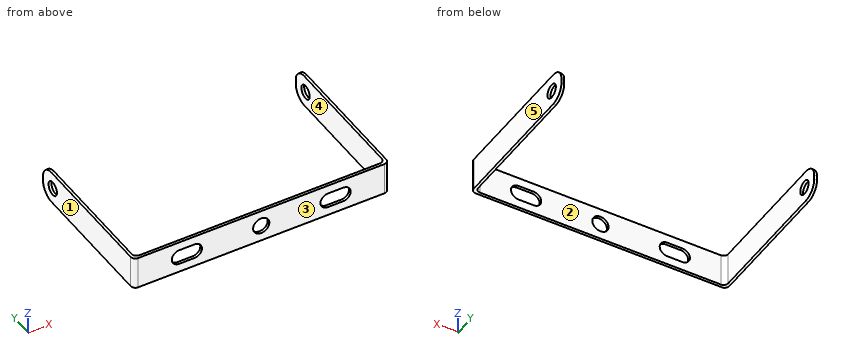
```python
from build123d import *

# Parameters (mm, degrees)
AUFSATZ_LINEAR_AUSTRAGEN1_DEPTH = 14
VERRUNDUNG1_R                   = 2
SKIZZE2_R                       = 3
SCHNITT_LINEAR_AUSTRAGEN1_DEPTH = 129.534042183
VERRUNDUNG2_R                   = 6
SKIZZE3_R                       = 3.5
SCHNITT_LINEAR_AUSTRAGEN2_DEPTH = 129.534042183


with BuildPart() as part:
    # Skizze1 → Aufsatz-Linear austragen1 (new body)
    with BuildSketch(Plane.XY):
        Polygon((0, 0), (-110, 0), (-110, 65), (-108.8, 65), (-108.8, 1.2), (-1.2, 1.2), (-1.2, 65), (0, 65), align=None)
    extrude(amount=AUFSATZ_LINEAR_AUSTRAGEN1_DEPTH)

    # Verrundung1
    verrundung1_edges = [part.edges().sort_by_distance(p)[0] for p in [
        (0, 0, 7),
        (-110, 0, 7),
        (-108.8, 1.2, 7),
        (-1.2, 1.2, 7),
    ]]
    fillet(verrundung1_edges, radius=VERRUNDUNG1_R)

    # Skizze2 → Schnitt-Linear austragen1 (cut, through all)
    with BuildSketch(Plane(origin=(0, 0, 0), x_dir=(0, 0, -1), z_dir=(1, 0, 0))):
        with Locations((-7, 58)):
            Circle(SKIZZE2_R)
    extrude(amount=-SCHNITT_LINEAR_AUSTRAGEN1_DEPTH, mode=Mode.SUBTRACT)

    # Verrundung2
    verrundung2_edges = [part.edges().sort_by_distance(p)[0] for p in [
        (-0.6, 65, 0),
        (-109.4, 65, 14),
        (-0.6, 65, 14),
        (-109.4, 65, 0),
    ]]
    fillet(verrundung2_edges, radius=VERRUNDUNG2_R)

    # Skizze3 → Schnitt-Linear austragen2 (cut, through all)
    with BuildSketch(Plane(origin=(0, 0, 0), x_dir=(-1, 0, 0), z_dir=(0, -1, 0))):
        with Locations(Location((55, -7, 0), (0, 0, 90))):
            Circle(SKIZZE3_R)
        with BuildLine():
            Line((90.25, -10.25), (83.75, -10.25))
            ThreePointArc((83.75, -10.25), (80.5, -7), (83.75, -3.75))
            Line((83.75, -3.75), (90.25, -3.75))
            ThreePointArc((90.25, -3.75), (93.5, -7), (90.25, -10.25))
        make_face()
        with BuildLine():
            Line((19.75, -10.25), (26.25, -10.25))
            ThreePointArc((26.25, -10.25), (29.5, -7), (26.25, -3.75))
            Line((26.25, -3.75), (19.75, -3.75))
            ThreePointArc((19.75, -3.75), (16.5, -7), (19.75, -10.25))
        make_face()
    extrude(amount=-SCHNITT_LINEAR_AUSTRAGEN2_DEPTH, mode=Mode.SUBTRACT)


solid = part.part
```
Verification items for the finished model (mm, model axes). Face numbers are marked on the shaded views. A direction names the side the tool comes from. Round coordinates to 2 decimals unless told otherwise and drop trailing zeros. Write each loop counter-clockwise with the first axis right and the second up, starting at its lowest first coordinate (ties: lowest second). Pieces come first, ordered by that corner, then holes.
1. Gauge pin test, flat ends, axial feed: P1, Ø7, axis at x = -78, z = 6, coming from the +Y side; P2, Ø5.5, axis at x = -55, z = 7, coming from the +Y side. Record the tip position at first contact, or that the pin passes through.
2. Draft check along X on the marked faces 3, 4 and 5. Enter one of: +X half, -X half, draft (parallel to the pull), parting line (faces both ways), or undercut.
3. Section check C-C on z = 12.5. Enter the section's corners in (x, y), plus the area to 3 significant figures.
4. Access from +Z, -Z, +X, -X, +Y, -Y to the whole of each face (thin tool, end or side, straight path). Record for the marked faces 1 and 2.
5. Section check D-D on z = 2. Enter the section's corners in (x, y), plus the area to 3 significant figures.
6. Scan lines: L1, parallel to X at y = 54, z = 1.25; L2, parallel to Y at x = -56, z = 12.5; L3, parallel to Y at x = -109.65, z = 7. Record each from-to range of solid material in increasing order.
7. Section check A-A on x = -55. Enter the section's corners in (y, z).
8. Section check B-B on y = 13. Enter the section's corners in (x, z), plus the area to 3 significant figures.
Answer:
1. P1: stops at y = 1.2
1. P2: passes through
2. face 3: draft
2. face 4: undercut
2. face 5: +X half
3. outline: (-110, 2) arc R2 ccw to (-108, 0) - (-2, 0) arc R2 ccw to (0, 2) - (0, 62.97) - (-1.2, 62.97) - (-1.2, 3.2) arc R2 cw to (-3.2, 1.2) - (-106.8, 1.2) arc R2 cw to (-108.8, 3.2) - (-108.8, 62.97) - (-110, 62.97) - close
3. area: 280 mm2
4. face 1: +Z, -Z, -X, +Y, -Y
4. face 2: +Z, -Z, +Y
5. outline: (-110, 2) arc R2 ccw to (-108, 0) - (-2, 0) arc R2 ccw to (0, 2) - (0, 63.47) - (-1.2, 63.47) - (-1.2, 3.2) arc R2 cw to (-3.2, 1.2) - (-106.8, 1.2) arc R2 cw to (-108.8, 3.2) - (-108.8, 63.47) - (-110, 63.47) - close
5. area: 281 mm2
6. L1: x = -110 to -108.8, -1.2 to 0
6. L2: y = 0 to 1.2
6. L3: y = 0.87 to 55, 61 to 65
7. outline: (0, 0) - (1.2, 0) - (1.2, 3.5) - (0, 3.5) - close; (0, 10.5) - (1.2, 10.5) - (1.2, 14) - (0, 14) - close
8. outline: (-110, 0) - (-108.8, 0) - (-108.8, 14) - (-110, 14) - close; (-1.2, 0) - (0, 0) - (0, 14) - (-1.2, 14) - close
8. area: 33.6 mm2
